Here's how the part is built. I have some questions about the finished solid (model axes, mm). Face numbers are marked on the shaded views. A direction names the side the tool comes from. Coordinates: 2 decimals unless noted, no trailing zeros. Write each loop counter-clockwise with the first axis right and the second up, starting at its lowest first coordinate (ties: lowest second). Pieces come first, ordered by that corner, then holes. Notation, with made-up numbers: (3.5, -24.75) -> (14.5, -24.75) arc R21 ccw to (14.5, -9.75) -> close; hole circle Ø7 at (36.25, -0.5). An arc over 180 degrees is marked (long way). Use a Markdown table: item, result. Add a question column.
Autodesk Inventor part; units mm, degrees
ref_plane "Work Plane2" through (0, 0, -24.5872) normal (0, 0, 1) x (1, 0, 0)
ref_plane "Work Plane5" through (4.5827, 33.4505, 7.9375) normal (0, 1, 0) x (0.5, 0, -0.866)
ref_plane "Work Plane6" through (0, 0, 32.766) normal (0, 0, 1) x (1, 0, 0)
sketch "Sketch3" plane through (0, 0, 0) normal (0, 1, 0) x (-1, 0, 0)
  circle A0 centre (0, 0) radius 10.7569
  dimension "d16" = 21.5138
extrude "Extrusion3" add sketch "Sketch3" along normal blind 26.67
sketch "Sketch4" plane through (0, 26.67, 0) normal (0, 1, 0) x (1, 0, 0)
  circle A0 centre (0, 0) radius 10.7569
  circle A1 centre (0, 0) radius 4.6101
  dimension "d19" = 9.2202
extrude "Extrusion4" add sketch "Sketch4" along normal blind 0.7137 contours A1
sketch "Sketch5" plane through (0, 27.3837, 0) normal (0, 1, 0) x (1, 0, 0)
  circle A0 centre (0, 0) radius 4.6101
  circle A1 centre (0, 0) radius 6.1468
  dimension "d22" = 12.2936
extrude "Extrusion5" add sketch "Sketch5" along normal blind 1.4275 contours A0 | A1
sketch "Sketch6" plane through (0, 28.8112, 0) normal (0, 1, 0) x (1, 0, 0)
  circle A0 centre (0, 0) radius 6.1468
  circle A1 centre (0, 0) radius 2.4587
  dimension "d25" = 4.9174
extrude "Extrusion6" add sketch "Sketch6" along normal mid plane 14.2748 contours A1
sketch "Sketch7" plane through (0, 35.9486, 0) normal (0, 1, 0) x (1, 0, 0)
  circle A0 centre (0, 0) radius 2.4587
  line L0 (9.1654, 0) -> (4.5827, -7.9375)
  line L1 (4.5827, -7.9375) -> (-4.5827, -7.9375)
  line L2 (-4.5827, -7.9375) -> (-9.1654, 0)
  line L3 (-9.1654, 0) -> (-4.5827, 7.9375)
  line L4 (-4.5827, 7.9375) -> (4.5827, 7.9375)
  line L5 (4.5827, 7.9375) -> (9.1654, 0)
  dimension "d28" = 15.875
extrude "Extrusion7" add sketch "Sketch7" against normal blind 4.9962 contours A0 | L0 L1 L2 L3 L4 L5
sketch "Sketch8" plane through (0, 0, 0) normal (1, 0, 0) x (0, 1, 0)
  line L0 (30.9524, 7.9375) -> (30.9524, 0)
  line L1 (30.9524, 8.6055) -> (30.9524, -7.9908)
  line L2 (30.9524, -7.9908) -> (54.6665, -21.6822)
  line L3 (54.6665, -21.6822) -> (54.6665, -100.584)
  line L4 (51.0978, -100.584) -> (51.0978, -23.7426)
  line L5 (51.0978, -23.7426) -> (27.3837, -10.0512)
  line L6 (27.3837, -10.0512) -> (27.3837, 8.6055)
  line L7 (54.6665, -100.584) -> (51.0978, -100.584)
  line L8 (30.9524, 8.6055) -> (27.3837, 8.6055)
  line L9 (35.9486, 0) -> (30.9524, 0)
  line L10 (0, 10.7569) -> (0, -10.7569)
  dimension "d31" = 3.5687
  dimension "d32" = 8.6055
  dimension "d33" = 120
  dimension "d34" = 100.584
  dimension "d36" = 7.9908
  dimension "d54" = 54.6665
extrude "Extrusion8" add sketch "Sketch8" along normal mid plane 10.0584
sketch "Sketch9" plane through (0, 26.67, 0) normal (0, 1, 0) x (1, 0, 0)
  circle A0 centre (0, 0) radius 10.7569
  line L0 (0, -10.7569) -> (0, 1.5367)
  line L1 (0, 1.5367) -> (-10.6466, 1.5367)
  circle A1 centre (0, 0) radius 4.6101
  dimension "d73" = 12.2936
extrude "Extrusion9" cut sketch "Sketch9" against normal blind 5.7099 contours L1 A1 L0 A0 | L1 L0 A1 picked at (-1.2328, -8.5574) picked at (-0.3635, -2.5175)
ref_plane "Work Plane2" through (0, 0, -24.5872) normal (0, 0, 1) x (1, 0, 0)
sketch "Sketch15" plane through (-5.0292, 27.3837, 8.6055) normal (0, -1, 0) x (1, 0, 0)
  line L0 (10.0584, 0) -> (0, 0)
  line L1 (5.0292, 0) -> (3.4925, 0)
  line L2 (3.4925, 0) -> (3.4925, -2.1514)
  line L3 (3.4925, -2.1514) -> (5.0292, -2.1514)
  line L4 (5.0292, 0) -> (5.0292, -2.1514)
  line L5 (5.0292, -131.4577) -> (5.0292, 24.4196)
  dimension "d63" = 2.1514
  dimension "d74" = 1.5367
extrude "Extrusion15" add sketch "Sketch15" along normal blind 5.7099
sketch "Sketch16" plane through (0, 0, 0) normal (0, 1, 0) x (-1, 0, 0)
  circle A0 centre (0, 0) radius 2.0625
extrude "Extrusion16" add sketch "Sketch16" along normal blind 28.5496
sketch "Sketch20" plane through (0, 0, 0) normal (1, 0, 0) x (0, 1, 0)
  line L0 (35.9486, 7.9375) -> (30.9524, 7.9375)
  line L1 (35.9486, 7.9375) -> (35.9486, 9.365)
  line L2 (35.9486, 9.365) -> (35.283, 9.365)
  line L3 (35.283, 9.365) -> (35.9486, 7.9375)
  line L4 (-7.1897, 0) -> (43.1383, 0)
  dimension "d94" = 1.4275
  dimension "d95" = 25
ref_plane "Work Plane5" through (4.5827, 33.4505, 7.9375) normal (0, 1, 0) x (0.5, 0, -0.866)
revolve "Revolution3" cut sketch "Sketch20" angle 360 about axis through (0, -10, 0) along (0, 1, 0)
ref_plane "Work Plane6" through (0, 0, 32.766) normal (0, 0, 1) x (1, 0, 0)
ref_plane "Work Plane9" through (0, 0, 32.766) normal (0, 0, 1) x (1, 0, 0)
sketch "Sketch29" plane through (0, 0, 32.766) normal (0, 0, 1) x (1, 0, 0)
  line L0 (0, 19.2474) -> (16.6688, 9.6237)
  line L1 (16.6688, 9.6237) -> (16.6688, -9.6237)
  line L2 (16.6688, -9.6237) -> (0, -19.2474)
  line L3 (0, -19.2474) -> (-16.6687, -9.6237)
  line L4 (-16.6687, -9.6237) -> (-16.6688, 9.6237)
  line L5 (-16.6688, 9.6237) -> (0, 19.2474)
  point P0 (0, 0)
  point P1 (0, 0)
  point P2 (16.6687, 0)
  dimension "d140" = 33.3375
extrude "Extrusion23" add sketch "Sketch29" against normal blind 9.2202
sketch "Sketch30" plane through (0, 0, 23.5458) normal (0, 0, -1) x (-1, 0, 0)
  line L0 (16.6688, 9.6237) -> (16.6687, -9.6237)
  line L1 (0, 19.2474) -> (0, -19.2474)
  circle A0 centre (0, 0) radius 19.2474
extrude "Extrusion24" add sketch "Sketch30" along normal blind 39.9542
sketch "Sketch31" plane through (0, 0, -16.4084) normal (0, 0, -1) x (-1, 0, 0)
  circle A0 centre (0, 0) radius 19.2474
  line L0 (0, 18.3309) -> (15.875, 9.1654)
  line L1 (15.875, 9.1654) -> (15.875, -9.1654)
  line L2 (15.875, -9.1654) -> (0, -18.3309)
  line L3 (0, -18.3309) -> (-15.875, -9.1654)
  line L4 (-15.875, -9.1654) -> (-15.875, 9.1654)
  line L5 (-15.875, 9.1654) -> (0, 18.3309)
  point P0 (-15.875, 0)
  dimension "d145" = 31.75
extrude "Extrusion25" add sketch "Sketch31" along normal blind 15.367 contours L0 L1 L2 L3 L4 L5
hole "Hole4" at (0, 0, 32.766) direction (0, 0, -1) diameter 21.7488 depth 18.4404
hole "Hole5" at (0, 0, -31.7754) direction (0, 0, 1) diameter 21.7488 depth 18.4404
hole "Hole6" at (0, 0, 14.3256) direction (0, 0, -1) diameter 17.399 end through all
sketch "Sketch32" plane through (0, 0, 0) normal (0, 1, 0) x (-1, 0, 0)
  line L0 (16.6688, 32.766) -> (0, 32.766)
  line L1 (16.6688, 32.766) -> (24.6063, 32.766)
  line L2 (24.6063, 32.766) -> (24.6063, 29.0647)
  line L3 (24.6063, 29.0647) -> (16.6688, 32.766)
  line L4 (0, -6.5532) -> (0, 39.3192)
  dimension "d157" = 25
  dimension "d158" = 7.9375
revolve "Revolution6" cut sketch "Sketch32" angle 360 about axis through (0, 0, -10) along (0, 0, 1)
sketch "Sketch33" plane through (0, 0, 0) normal (0, 1, 0) x (-1, 0, 0)
  line L0 (0, -31.7754) -> (15.875, -31.7754)
  line L1 (15.875, -31.7754) -> (0, -31.7754)
  line L2 (0, -16.4084) -> (0, -31.7754)
  line L3 (15.875, -16.4084) -> (15.875, -31.7754)
  line L4 (15.875, -31.7754) -> (23.8125, -31.7754)
  line L5 (23.8125, -31.7754) -> (23.8125, -28.0741)
  line L6 (23.8125, -28.0741) -> (15.875, -31.7754)
  line L7 (0, -38.1305) -> (0, 6.3551)
  line L8 (15.875, -16.4084) -> (0, -16.4084)
  point P0 (0, -17.3736)
  dimension "d160" = 25
  dimension "d161" = 7.9375
revolve "Revolution7" cut sketch "Sketch33" angle 360 about axis through (0, 0, -10) along (0, 0, 1) contours L6 L5 L4
sketch "Sketch34" plane through (5.0292, 51.0978, -100.584) normal (0, 0, -1) x (-1, 0, 0)
  line L0 (0, 3.5687) -> (0, 0)
  line L1 (0, 3.5687) -> (10.0584, 3.5687)
  line L2 (-0.7544, 4.4012) -> (10.8128, 4.4012)
  line L3 (10.8128, 4.4012) -> (10.8128, -0.628)
  line L4 (10.8128, -0.628) -> (-0.7544, -0.628)
  line L5 (-0.7544, -0.628) -> (-0.7544, 4.4012)
  point P0 (0, 1.7843)
  point P1 (-0.7544, 1.8866)
  point P2 (5.0292, 3.5687)
  point P3 (5.0292, 4.4012)
  point P4 (5.0292, -51.0978)
  dimension "d163" = 11.5672
  dimension "d164" = 5.0292
  dimension "d165" = 55.499
extrude "Extrusion26" add sketch "Sketch34" against normal blind 70.4088
thread "Thread4"
thread "Thread5"
equation "\"d16\" = 0.35 * M"
equation "\"d17\" = 0.8 * C_HEX"
equation "\"d19\" = 0.15 * M"
equation "\"d20\" = 0.01 * N1"
equation "\"d22\" = 0.2 * M"
equation "\"d23\" = 0.02 * N1"
equation "\"d25\" = 0.08 * M"
equation "\"d26\" = 0.2 * N1"
equation "\"d28\" = 0.5 * B_HEX"
equation "\"d29\" = 0.07 * N1"
equation "\"d31\" = 0.05 * N1"
equation "\"d32\" = 0.14 * M"
equation "\"d34\" = H1"
equation "\"d36\" = 0.13 * M"
equation "\"d54\" = -0.4925 * B_HEX + 0.985 * N1"
equation "\"d37\" = 0.1 * H1"
equation "\"d73\" = 0.2 * M"
equation "\"d39\" = 0.08 * N1"
equation "\"d63\" = 0.035 * M"
equation "\"d74\" = 0.025 * M"
equation "\"d64\" = 0.08 * N1"
equation "\"d75\" = 0.4 * N1"
equation "\"d94\" = 0.02 * N1"
equation "\"d140\" = C_HEX"
equation "\"d141\" = 0.15 * M"
equation "\"d143\" = 0.65 * M"
equation "\"d145\" = B_HEX"
equation "\"d146\" = 0.25 * M"
equation "\"d150\" = 1.25 * D"
equation "\"d155\" = 0.3 * M"
equation "\"d178\" = d150"
equation "\"d183\" = 0.3 * M"
equation "\"d187\" = D"
equation "\"d192\" = 0.3 * M"
equation "\"d158\" = 0.25 * B_HEX"
equation "\"d161\" = 0.25 * B_HEX"
equation "\"d163\" = 0.115 * H1"
equation "\"d164\" = 0.05 * H1"
equation "\"d166\" = 0.7 * H1"
equation "\"d170\" = 0.2 * M"
equation "\"d172\" = 0.2 * M"
equation "\"D\" = 17.399"
equation "\"N1\" = 71.374"
equation "\"M\" = 61.468"
equation "\"H1\" = 100.584"
equation "\"L\" = 133.35"
equation "\"B_HEX\" = 31.75"
equation "\"C_HEX\" = 33.3375"
equation "\"d41\" = -0.4 * M"
equation "\"d104\" = L - H1"
equation "\"d139\" = L - H1"
equation "\"P_TH\" = 6.35"
equation "\"Parker_No\" = 1.2345"
properties part number "Parker Female-Female Pipe Ends XV500P XV500P-12" material "Brass, Soft Yellow"
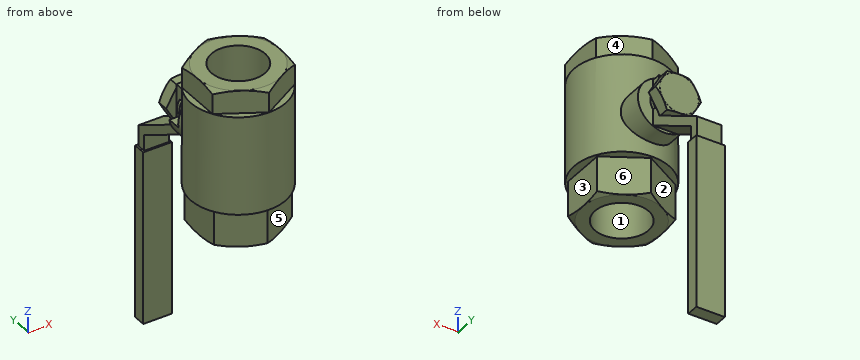
Q1. Which directions (+Z, -Z, +X, -X, +Y, -Y) give clear straight access to the entire face, cutting with the end or side of a thin tool? Please do the marked faces 4, 5 and 6.
Q2. Suppose I cut it at B-B, the plane y = 24. Write out the boundary of the cut face in (x, z) (1 decimal), and give its area (3 significant figures).
Q3. Suppose I cut it at A-A, the plane z = -26.5. Write out the boundary of the cut face in (x, y) (1 decimal), and give its area (3 significant figures).
Q4. Suppose I cut it at C-C, the plane z = 19. Write out the boundary of the cut face in (x, y).
Q5. Thinking about a two-plate mould opening in X: for the marked faces 1, 2 and 3, which applies, released by +X, released by -X, zero draft, split by the parting line, or undercut?
Q6. Please list where these lines run through material, in increasing order: line 1 (Y direction, x = 0, z = 1.75); line 2 (X direction, y = 0, z = 1.25); line 3 (X direction, y = 0, z = 23).
Q7. Will these pins go through, and if not, where does the flat tip stop? pin 1 (5.5 mm diameter, centred on x = -1, y = 33.5, fed in from +Z); pin 2 (5 mm diameter, centred on x = -2.5, z = -46.5, fed in from -Y); pin 3 (0.5 mm diameter, centred on x = -0.5, y = 26, fed in from -Z); pin 4 (6.5 mm diameter, centred on x = -2.5, y = -3.5, fed in from -Z) (3 decimals).
Answer key:
| question | item | result |
|---|---|---|
| 1 | face 4 | +Z, +X, +Y |
| 1 | face 5 | -Z, +X, -Y |
| 1 | face 6 | -Z, +X |
| 2 | outline | (-10.6, -1.5) arc R10.8 ccw (long way) to (0, 10.8) -> (0, 8.6) -> (-1.5, 8.6) -> (-1.5, 6.5) -> (0, 6.5) -> (0, 2.1) arc R2.1 ccw to (-1.4, -1.5) -> close |
| 2 | area | 266 mm^2 |
| 3 | outline | (-15.9, -9.2) -> (0, -18.3) -> (15.9, -9.2) -> (15.9, 9.2) -> (0, 18.3) -> (-15.9, 9.2) -> close; (-5, 51.1) -> (5, 51.1) -> (5, 54.7) -> (-5, 54.7) -> close; hole circle Ø21.7 at (0, 0) |
| 3 | area | 537 mm^2 |
| 4 | outline | circle Ø38.49 at (0, 0); hole circle Ø21.75 at (0, 0) |
| 5 | face 1 | undercut |
| 5 | face 2 | released by -X |
| 5 | face 3 | released by +X |
| 6 | line 1 | y = -19.25 to -8.7, 8.7 to 35.95 |
| 6 | line 2 | x = -19.25 to -8.7, 8.7 to 19.25 |
| 6 | line 3 | x = -19.25 to -10.87, 10.87 to 19.25 |
| 7 | pin 1 | stops at z = 8.61 |
| 7 | pin 2 | stops at y = 50.47 |
| 7 | pin 3 | stops at z = -10.75 |
| 7 | pin 4 | passes through |
